Geometry: see drawing. Coordinates: mm, zero at the bounding-box minimum. Round coordinates to 2 decimals unless told otherwise and drop trailing zeros. Write each loop counter-clockwise with the first axis right and the second up, starting at its lowest first coordinate (ties: lowest second). Pieces come first, ordered by that corner, then holes. Notation, with made-up numbers: (-1.5, 85.25) -> (17.5, 85.25) arc R18 cw to (17.5, 113.25) -> close; hole circle Ø6 at (75, -23.75). An arc over 180 degrees is marked (long way). Write item = value, one per line.
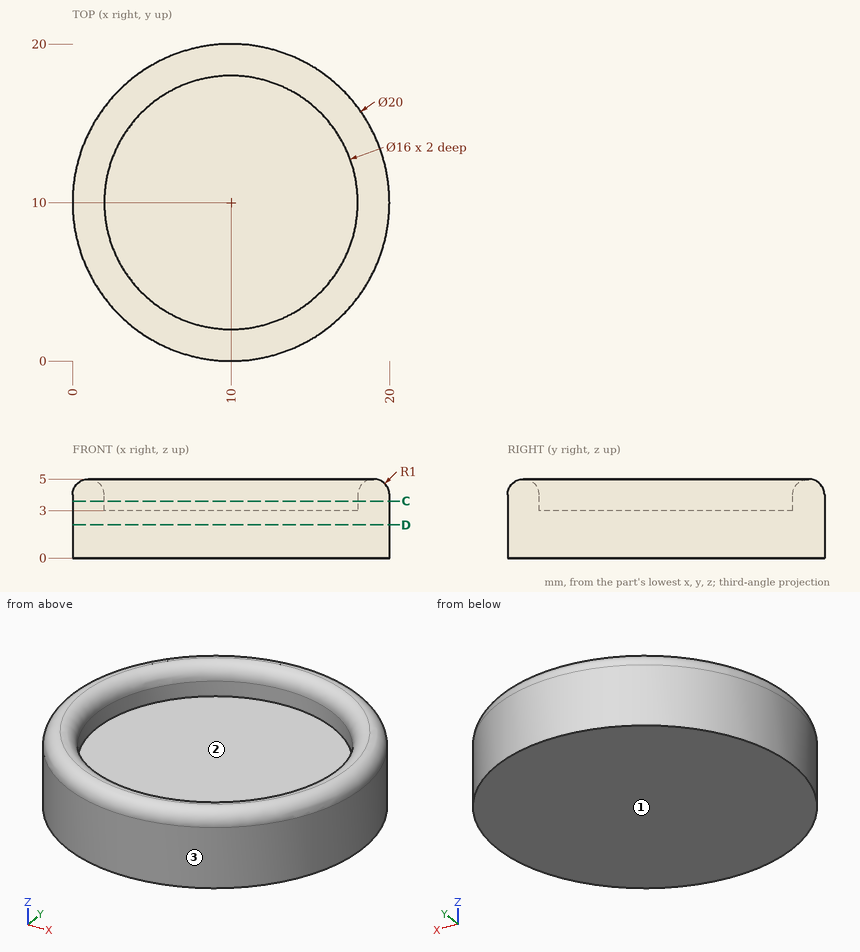
1) Draft query along Y for the marked faces 1, 2 and 3. Return one class per face: +Y half, -Y half, draft (parallel to the pull), parting line (faces both ways), or undercut.
Solutions:
face_1 = draft
face_2 = undercut
face_3 = parting line
2) Line query: L1, parallel to Y at x = 10, z = 3.35; L2, parallel to Z at x = 7.5, y = 15.25; L3, parallel to X at y = 3.25, z = 3.6. Output: solid intervals per line, ascending. Write a range as from..to.
Solutions:
L1 = 0..2, 18..20
L2 = 0..3
L3 = 2.62..5.71, 14.29..17.38
3) First-contact query: P1, Ø1, axis at y = 9, z = 0.5, coming from the +X side; P2, Ø1.5, axis at y = 15, z = 3, coming from the -X side; P3, Ø1.5, axis at y = 2, z = 4.5, coming from the +X side. Flat tips, straight axial feed; report the tip coordinate or a pass-through.
Solutions:
P1 = 19.99
P2 = 0.95
P3 = 16.8
4) Cut plane D-D (z = 2.1). Return the cut outline in (x, y).
Solutions:
outline = circle Ø20 at (10, 10)
5) Cut plane C-C (z = 3.6). Return the cut outline in (x, y), and give its area (3 significant figures).
Solutions:
outline = circle Ø20 at (10, 10); hole circle Ø16 at (10, 10)
area = 113 mm^2
